Check sheet for the modelled part. Datum: model origin and axes. Units: mm. A direction names the side the tool comes from. Coordinates: 2 decimals unless noted, no trailing zeros. Loops run counter-clockwise (first coordinate to the right, second up) from the corner with the lowest first, then second, coordinate; pieces in that order, holes last. Notation, with made-up numbers: (77, -32) -> (104, -32) arc R15 cw to (104, -14) -> close; hole circle Ø10 at (12.5, 25). An arc over 180 degrees is marked (long way). Use CSV: the item, a comma, the result in double quotes. Start each with the question number.
1. Gauge pin test, flat ends, axial feed: pin 1 (1 mm diameter, centred on y = 20, z = 71, fed in from -X); pin 2 (4.5 mm diameter, centred on x = -11, y = -17, fed in from -Z); pin 3 (6.5 mm diameter, centred on y = -19, z = 6.5, fed in from +X); pin 4 (3 mm diameter, centred on x = -63.5, y = -8.5, fed in from -Z). Record the tip position at first contact, or that the pin passes through.
2. Sectioned sample at C-C, the plane z = 29. Record the cut outline in (x, y).
3. Sectioned sample at A-A, the plane y = 0. Record the cut outline in (x, z).
4. Sectioned sample at B-B, the plane x = -16. Record the cut outline in (y, z).
5. Sectioned sample at D-D, the plane y = 10.5. Record the cut outline in (x, z).
6. Release check for a two-part mould opening along Y. For faces 4 (the face through (-7, 9.291, 77)), 5 (the face through (-7, 18, 94.742)), 6 (the face through (-37, -27.021, 6)) record: pulls with the +Y half, pulls with the -Y half, needs draft (parallel to the pull), parting line crosses it, or undercut.
7. Thickness scan on L1, parallel to Y at x = -6, z = 64.5; L2, parallel to Z at x = -66, y = -8; L3, parallel to X at y = -12, z = 38.5. Record the ranges inside material, lowest first.
8. Set-up check for faces 1 (the face through (-13, -11.375, 8)), 2 (the face through (-7, -9.291, 77)), 3 (the face through (-26.416, -19, 6)): record each of +Z, -Z, +X, -X, +Y, -Y from which the full face is reachable in a straight line by a thin tool's end or side.
```python
from build123d import *

# Parameters (mm, degrees)
F1_DEPTH = 12.7
F2_W     = 14.5472725853
F2_H     = 54.0411157981
F3_DEPTH = 82.042
F5_DEPTH = 25.4
F6_W     = 15.6459464915
F6_H     = 20.0112983584
F7_DEPTH = 26.416


with BuildPart() as f1:
    # F0 (on Top) → F1 (new body)
    with BuildSketch(Plane.XY):
        with BuildLine():
            Line((0, 27.020557899), (-48.259999603, 27.020557899))
            ThreePointArc((-48.259999603, 27.020557899), (-75.2805575021, 0), (-48.259999603, -27.020557899))
            Line((-48.259999603, -27.020557899), (0, -27.020557899))
            Line((0, -27.020557899), (0, 27.020557899))
        make_face()
    extrude(amount=F1_DEPTH)

    # F2 (on face) → F3 (join)
    with BuildSketch(Plane.XY.offset(12.7)):
        with Locations((-7.2736362927, 0)):
            Rectangle(F2_W, F2_H)
    extrude(amount=F3_DEPTH)

    # F4 (on face) → F5 (cut)
    with BuildSketch(Plane(origin=(-14.5472725853, 0, 0), x_dir=(0, -1, 0), z_dir=(-1, 0, 0))):
        with BuildLine():
            Line((-9.2913275192, 94.742), (-9.2913275192, 59.2682287097))
            ThreePointArc((-9.2913275192, 59.2682287097), (0, 49.9769011905), (9.2913275192, 59.2682287097))
            Line((9.2913275192, 59.2682287097), (9.2913275192, 94.742))
            Line((9.2913275192, 94.742), (-9.2913275192, 94.742))
        make_face()
    extrude(amount=-F5_DEPTH, mode=Mode.SUBTRACT)

    # F6 (on face) → F7 (cut)
    with BuildSketch(Plane.YZ):
        with Locations((-19.1975846533, 10.0056491792)):
            Rectangle(F6_W, F6_H)
    extrude(amount=-F7_DEPTH, mode=Mode.SUBTRACT)


solid = f1.part
```
Completed:
1,pin 1,"x = -14.55"
1,pin 2,"z = 20.01"
1,pin 3,"x = -26.42"
1,pin 4,"z = 0"
2,outline,"(-14.55, -27.02) -> (0, -27.02) -> (0, 27.02) -> (-14.55, 27.02) -> close"
3,outline,"(-75.28, 0) -> (0, 0) -> (0, 49.98) -> (-14.55, 49.98) -> (-14.55, 12.7) -> (-75.28, 12.7) -> close"
4,outline,"(-11.37, 0) -> (27.02, 0) -> (27.02, 12.7) -> (-11.37, 12.7) -> close"
5,outline,"(-73.16, 0) -> (0, 0) -> (0, 94.74) -> (-14.55, 94.74) -> (-14.55, 12.7) -> (-73.16, 12.7) -> close"
6,face 4,"undercut"
6,face 5,"needs draft"
6,face 6,"pulls with the -Y half"
7,L1,"-27.02 to -9.29, 9.29 to 27.02"
7,L2,"0 to 12.7"
7,L3,"-14.55 to 0"
8,face 1,"-Z, +X, -Y"
8,face 2,"+Z, +X, -X"
8,face 3,"+Z, -Z, +X, -Y"
